from build123d import *

# Parameters (mm, degrees)
F0_R     = 5
F0_R_2   = 7.5
F1_DEPTH = 25


with BuildPart() as f1:
    # F0 (on Top) → F1 (new body)
    with BuildSketch(Plane.XY):
        with BuildLine():
            ThreePointArc((56.302521, -13.680972), (81.43664, -11.977341), (80.252101, 13.186585))
            ThreePointArc((80.252101, 13.186585), (34.639129, 29.041183), (-7.882353, 6.15374))
            ThreePointArc((-7.882353, 6.15374), (-7.576127, -6.527043), (4.919786, -8.706073))
            ThreePointArc((4.919786, -8.706073), (31.395464, -3.092849), (56.302521, -13.680972))
        make_face()
        Circle(F0_R, mode=Mode.SUBTRACT)
        with Locations((68, 0)):
            Circle(F0_R_2, mode=Mode.SUBTRACT)
        with BuildLine():
            ThreePointArc((44.950326, 0.142182), (29.540091, 3.306499), (13.896058, 1.647439))
            ThreePointArc((13.896058, 1.647439), (11.117549, 1.916957), (9.191943, 3.938043))
            ThreePointArc((9.191943, 3.938043), (8.380408, 5.456075), (7.320562, 6.812443))
            ThreePointArc((7.320562, 6.812443), (6.267781, 9.926776), (7.904024, 12.778113))
            ThreePointArc((7.904024, 12.778113), (30.530218, 22.242438), (55.005596, 20.669565))
            ThreePointArc((55.005596, 20.669565), (57.763559, 17.645265), (56.418739, 13.779492))
            ThreePointArc((56.418739, 13.779492), (52.422533, 9.019009), (50.283693, 3.183153))
            ThreePointArc((50.283693, 3.183153), (48.328016, 0.415678), (44.950326, 0.142182))
        make_face(mode=Mode.SUBTRACT)
    extrude(amount=F1_DEPTH)


solid = f1.part
Design review of the part built by this model. Coordinates are the model's own, in mm. A direction names the side the tool comes from. Coordinates: 2 decimals unless noted, no trailing zeros. Loops run counter-clockwise (first coordinate to the right, second up) from the corner with the lowest first, then second, coordinate; pieces in that order, holes last. Notation, with made-up numbers: (84.5, 88) -> (134.5, 88) arc R17 ccw to (134.5, 118) -> close; hole circle Ø9 at (-26.5, 73.25). An arc over 180 degrees is marked (long way). Use a Markdown table: item, result. Add a question column.
Item 1: Clearance check with flat-ended pins moving along their axes: P1, Ø2, axis at y = 5.5, z = 18, coming from the +X side; P2, Ø8, axis at x = 35, z = 18.5, coming from the -Y side; P3, Ø4, axis at x = 29, z = 11.5, coming from the -Y side. State where each tip first meets the part, or that it passes through.
Item 2: We need section B-B, the plane y = -6. Write out the cut boundary in (x, z).
Item 3: The part is to be moulded in two halves that separate along Y. For faces 3 (the cylindrical face through (81.17, -12.27, 12.32)), 4 (the cylindrical face through (29.761, 3.295, 12.325)), 5 (the flat face through (37, 1, 25)), say which applies: +Y half, -Y half, draft (parallel to the pull), parting line (faces both ways), or undercut.
Item 4: Machinability: for faces 1 (the cylindrical face through (35.333, 29.093, 12.325)), 2 (the cylindrical face through (48.37, 0.44, 12.32)), which of the approach directions +Z, -Z, +X, -X, +Y, -Y give a long, thin tool a straight path to every point of the face, cutting with its end or side? Answer none if there is none.
Item 5: Wall thickness on L1, parallel to Y at x = 32.5, z = 12; L2, parallel to X at y = 16, z = 22.5; L3, parallel to Y at x = 20, z = 18.5: over which ranges is each line inside the solid? List them lowest first. Write a range as from..to.
Item 6: We need section D-D, the plane x = 24.5. Write out the cut boundary in (y, z), and give its area (3 significant figures).
Item 7: We need section C-C, the plane z = 5. Write out the cut boundary in (x, y), and give its area (3 significant figures).
Item 8: We need section A-A, the plane x = 64.5. Write out the cut boundary in (y, z), and give its area (3 significant figures).
Numbers:
| question | item | result |
|---|---|---|
| 1 | P1 | stops at x = 85.43 |
| 1 | P2 | stops at y = -4.5 |
| 1 | P3 | stops at y = -3.06 |
| 2 | outline | (-8, 0) -> (10.6, 0) -> (10.6, 25) -> (-8, 25) -> close; (43.51, 0) -> (63.5, 0) -> (63.5, 25) -> (43.51, 25) -> close; (72.5, 0) -> (84.97, 0) -> (84.97, 25) -> (72.5, 25) -> close |
| 3 | face 3 | parting line |
| 3 | face 4 | undercut |
| 3 | face 5 | draft |
| 4 | face 1 | +Z, -Z, +Y |
| 4 | face 2 | +Z, -Z |
| 5 | L1 | y = -3.21..3.08, 22.54..28.83 |
| 5 | L2 | x = 1.83..12.92, 57.76..77 |
| 5 | L3 | y = -3.44..2.88, 19.35..26 |
| 6 | outline | (-2.96, 0) -> (3.3, 0) -> (3.3, 25) -> (-2.96, 25) -> close; (20.87, 0) -> (27.35, 0) -> (27.35, 25) -> (20.87, 25) -> close |
| 6 | area | 318 mm^2 |
| 7 | outline | (-7.88, 6.15) arc R10 ccw to (4.92, -8.71) arc R45 cw to (56.3, -13.68) arc R18 ccw to (80.25, 13.19) arc R60 ccw to start; hole circle Ø10 at (0, 0); hole (7.32, 6.81) arc R10 cw to (9.19, 3.94) arc R4 ccw to (13.9, 1.65) arc R51.25 cw to (44.95, 0.14) arc R4 ccw to (50.28, 3.18) arc R18 cw to (56.42, 13.78) arc R4 ccw to (55.01, 20.67) arc R53.75 ccw to (7.9, 12.78) arc R4 ccw to start; hole circle Ø15 at (68, 0) |
| 7 | area | 1,860 mm^2 |
| 8 | outline | (-17.66, 0) -> (-6.63, 0) -> (-6.63, 25) -> (-17.66, 25) -> close; (6.63, 0) -> (23.73, 0) -> (23.73, 25) -> (6.63, 25) -> close |
| 8 | area | 703 mm^2 |
